```python
from build123d import *

# Parameters (mm, degrees)
F0_W     = 9.525
F0_H     = 19.05
F0_R     = 2.15265
F1_DEPTH = 15.875
F2_W     = 9.525
F2_H     = 3.175
F3_DEPTH = 9.525
F4_R     = 2.15265
F5_DEPTH = 9.525


with BuildPart() as f1:
    # F0 (on Top) → F1 (new body)
    with BuildSketch(Plane.XY):
        with Locations((4.7625, 9.525)):
            Rectangle(F0_W, F0_H)
        with Locations((4.7625, 14.2875)):
            Circle(F0_R, mode=Mode.SUBTRACT)
    extrude(amount=F1_DEPTH)

    # F2 (on face) → F3 (cut)
    with BuildSketch(Plane(origin=(0, 19.05, 0), x_dir=(-1, 0, 0), z_dir=(0, 1, 0))):
        with Locations((-4.7625, 1.5875)):
            Rectangle(F2_W, F2_H)
        with Locations((-4.7625, 14.2875)):
            Rectangle(F2_W, F2_H)
    extrude(amount=-F3_DEPTH, mode=Mode.SUBTRACT)

    # F4 (on face) → F5 (cut, through all)
    with BuildSketch(Plane(origin=(0, 0, 0), x_dir=(0, -1, 0), z_dir=(-1, 0, 0))):
        with Locations((-4.7625, 7.9375)):
            Circle(F4_R)
    extrude(amount=-F5_DEPTH, mode=Mode.SUBTRACT)


solid = f1.part
```
Can you work these out from the model? Positions are in its coordinate system, mm. A direction names the side the tool comes from. Round coordinates to 2 decimals unless told otherwise and drop trailing zeros. Loops run counter-clockwise (first coordinate to the right, second up) from the corner with the lowest first, then second, coordinate; pieces in that order, holes last. Notation, with made-up numbers: M 77.5,14.5 L 125.5,14.5 A30 ccw 125.5,52.5 Z; hole C 56.5,41 d8. An arc over 180 degrees is marked long. Answer as a JSON object with one key per item and string values. Group by question number.
Q1. Imagine slicing it at A-A, the plane x = 3.75. Count the separate pieces of the cut face and the enclosed holes in it, then the cut area to 3 significant figures.
Q2. We'd pull the mould along X, two halves only. Please class faces 4 (the cylindrical face through (5.92, 16.103, 7.871)), 5 (the flat face through (5, 19.05, 8)), 6 (the flat face through (9.525, 7.3, 7.8)): +X half, -X half, draft (parallel to the pull), parting line (faces both ways), or undercut.
Q3. Imagine slicing it at C-C, the plane y = 6. Please give me the cut outline in (x, z) (3 decimals).
Q4. On a 3-axis mill with a long thin cutter (end or side, diameter ignored), from which of +Z, -Z, +X, -X, +Y, -Y can I reach the whole of each face in a straight line? I mean faces 1 (the flat face through (5, 0, 8)), 2 (the flat face through (5, 9.525, 14)), 3 (the flat face through (5, 9.525, 2)). Say none if no direction works.
Q5. Please list where these lines run through material, in increasing order: L1, parallel to Z at x = 2, y = 10 (3 decimals); L2, parallel to Y at x = 8, z = 1.75 (3 decimals); L3, parallel to Y at x = 4.5, z = 9.5.
Q6. Will these pins go through, and if not, where does the flat tip stop? pin 1 (5 mm diameter, centred on x = 5.5, y = 16.5, fed in from -Z) (3 decimals); pin 2 (1.5 mm diameter, centred on x = 1.5, y = 15, fed in from +Z).
Findings:
{
 "1": {"separate pieces": "2", "enclosed holes": "1", "area": "191 mm2"},
 "2": {"face 4": "undercut", "face 5": "draft", "face 6": "+X half"},
 "3": {"outline": "M 0,0 L 9.525,0 L 9.525,6.176 L 0,6.176 Z; M 0,9.699 L 9.525,9.699 L 9.525,15.875 L 0,15.875 Z"},
 "4": {"face 1": "+Z, -Z, +X, -X, -Y", "face 2": "+Z, +X, -X, +Y", "face 3": "-Z, +X, -X, +Y"},
 "5": {"L1": "z = 3.175 to 12.7", "L2": "y = 0 to 9.525", "L3": "y = 0 to 3.28, 6.24 to 12.15, 16.42 to 19.05"},
 "6": {"pin 1": "stops at z = 3.175", "pin 2": "stops at z = 12.7"}
}
